The listing builds one solid part. Answer for the finished solid, in the listing's coordinates (mm). Face numbers are marked on the shaded views. A direction names the side the tool comes from. Give positions to 0.01 mm unless a question says otherwise; leave off trailing zeros. Order: outer loops, then holes, each group sorted by start corner. A loop starts at its lowest first (then second) coordinate and runs counter-clockwise, first axis right, second up. Notation, with made-up numbers: (-19.75, -11.75) - (16.25, -11.75) arc R20 cw to (16.25, -6.75) - close; hole circle Ø4 at (-21.5, -21). An arc over 180 degrees is marked (long way). Use a Markdown table: item, result. Add a question column.
1) Find section A-A, the plane x = 44. Determine the outline of the cut face in (y, z), plus the area to 3 significant figures.
2) Find section C-C, the plane z = -59.5. Determine the outline of the cut face in (x, y).
3) The mould has two halves that part along Z. Classify the marked faces 4, 5 and 6: released by +Z, released by -Z, zero draft, split by the parting line, or undercut.
4) Find section B-B, the plane y = 3. Determine the outline of the cut face in (x, z), plus the area to 3 significant figures.
5) For the marked faces 1, 2 and 3, determine the directions among +Z, -Z, +X, -X, +Y, -Y from which every point of the face is accessible in a straight line to the end or side of a thin tool.
6) Find section D-D, the plane x = 22.5. Determine the outline of the cut face in (y, z).
7) Straight lines are drawn through the part: line 1 (X direction, y = 12.5, z = -70); line 2 (Z direction, x = 44.5, y = 5); line 3 (X direction, y = 2.5, z = -29). For each, find the intervals that lie inside material, in ascending order.
8) Flat-ended cylindrical pins translate along their axes: pin 1 (3 mm diameter, centred on x = 25.5, y = 28, fed in from -Z); pin 2 (6 mm diameter, centred on x = 29, z = -21.5, fed in from +Y); pin 3 (3 mm diameter, centred on x = 31, y = 15, fed in from -Z); pin 4 (2 mm diameter, centred on y = 12.5, z = -39, fed in from +X). Find the tip coordinate at first contact, or state that the pin passes through.
from build123d import *

# Parameters (mm, degrees)
BOSS_EXTRUDE1_DEPTH = 12
BOSS_EXTRUDE3_DEPTH = 25


with BuildPart() as part:
    # Sketch1 → Boss-Extrude1 (new body)
    with BuildSketch(Plane(origin=(0, 0, 0), x_dir=(1, 0, 0), z_dir=(0, 1, 0))):
        Polygon((0, 0), (0, 75), (50, 75), (50, 50), (38, 50), (38, 25), (50, 25), (50, 0), align=None)
    extrude(amount=BOSS_EXTRUDE1_DEPTH)

    # Sketch6 → Boss-Extrude3 (add)
    with BuildSketch(Plane.ZY):
        Polygon((-55, 32), (-20, 12), (-55, 12), (-75, 12), (-75, 32), align=None)
    extrude(amount=-BOSS_EXTRUDE3_DEPTH)


solid = part.part
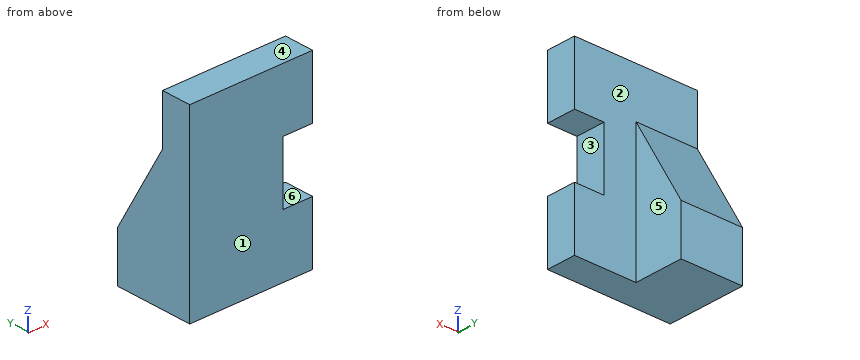
The answers:
| question | item | result |
|---|---|---|
| 1 | outline | (0, -75) - (12, -75) - (12, -50) - (0, -50) - close; (0, -25) - (12, -25) - (12, 0) - (0, 0) - close |
| 1 | area | 600 mm2 |
| 2 | outline | (0, 0) - (50, 0) - (50, 12) - (25, 12) - (25, 32) - (0, 32) - close |
| 3 | face 4 | released by +Z |
| 3 | face 5 | zero draft |
| 3 | face 6 | undercut |
| 4 | outline | (0, -75) - (50, -75) - (50, -50) - (38, -50) - (38, -25) - (50, -25) - (50, 0) - (0, 0) - close |
| 4 | area | 3,450 mm2 |
| 5 | face 1 | +Z, -Z, +X, -X, -Y |
| 5 | face 2 | +Z, +X, +Y |
| 5 | face 3 | +X, +Y, -Y |
| 6 | outline | (0, -75) - (32, -75) - (32, -55) - (12, -20) - (12, 0) - (0, 0) - close |
| 7 | line 1 | 0 to 25 |
| 7 | line 2 | -75 to -50, -25 to 0 |
| 7 | line 3 | 0 to 38 |
| 8 | pin 1 | z = -75 |
| 8 | pin 2 | y = 12 |
| 8 | pin 3 | through |
| 8 | pin 4 | x = 38 |
